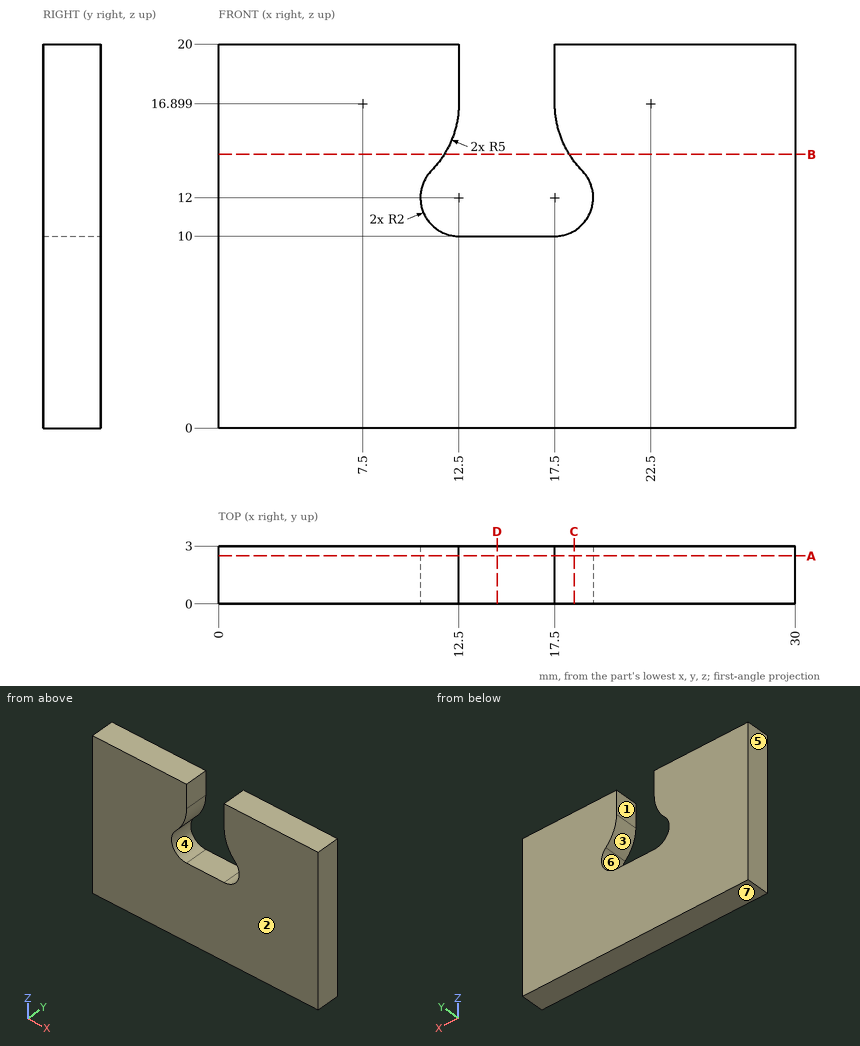
Print and shaded views of the part. All mm, measured from the part's lowest x, y and z. A direction names the side the tool comes from. Round coordinates to 2 decimals unless told otherwise and drop trailing zeros. Write each loop counter-clockwise with the first axis right and the second up, starting at its lowest first coordinate (ties: lowest second). Pieces come first, ordered by that corner, then holes. Notation, with made-up numbers: (2.5, -34) -> (12.5, -34) arc R24 cw to (12.5, -6) -> close; hole circle Ø10 at (39, 69.5). An arc over 180 degrees is marked (long way). Return JSON: item names as keys, results as strings. Group by question number.
Q1. Saw through at C-C on x = 18.5. Write the cut outline in (y, z), plus the area to 3 significant figures.
Q2. Pin check, flat tip, straight feed: pin 1 (4 mm diameter, centred on x = 13.5, z = 5, fed in from -Y). Stop position of the tip, or through.
Q3. Probe L1, parallel to X at y = 2.95, z = 18; L2, parallel to Z at x = 15.5, y = 2.3; L3, parallel to X at y = 1.4, z = 14.5. List the from-to ranges inside material, lowest first. Write a range as [from, to].
Q4. Saw through at D-D on x = 14.5. Write the cut outline in (y, z).
Q5. Mould opens along X. For the marked faces 4, 5, 6 and 7 say: pulls with the +X half, pulls with the -X half, needs draft (parallel to the pull), parting line crosses it, or undercut.
Q6. Saw through at A-A on y = 2.5. Write the cut outline in (x, z).
Q7. Which spindle directions (+Z, -Z, +X, -X, +Y, -Y) get a long thin tool onto all of the face, cutting with end or side? Do the marked faces 1, 2 and 3. Say none if no direction does.
Q8. Saw through at B-B on z = 14.25. Write the cut outline in (x, y), plus the area to 3 significant figures.
Answer:
{
 "1": {"outline": "(0, 0) -> (3, 0) -> (3, 10.27) -> (0, 10.27) -> close; (0, 13.9) -> (3, 13.9) -> (3, 20) -> (0, 20) -> close", "area": "49.1 mm2"},
 "2": {"pin 1": "y = 0"},
 "3": {"L1": "[0, 12.5], [17.5, 30]", "L2": "[0, 10]", "L3": "[0, 11.89], [18.11, 30]"},
 "4": {"outline": "(0, 0) -> (3, 0) -> (3, 10) -> (0, 10) -> close"},
 "5": {"face 4": "undercut", "face 5": "pulls with the -X half", "face 6": "undercut", "face 7": "needs draft"},
 "6": {"outline": "(0, 0) -> (30, 0) -> (30, 20) -> (17.5, 20) -> (17.5, 16.9) arc R5 ccw to (18.93, 13.4) arc R2 cw to (17.5, 10) -> (12.5, 10) arc R2 cw to (11.07, 13.4) arc R5 ccw to (12.5, 16.9) -> (12.5, 20) -> (0, 20) -> close"},
 "7": {"face 1": "+Z, +Y, -Y", "face 2": "+Z, -Z, +X, -X, -Y", "face 3": "+Y, -Y"},
 "8": {"outline": "(0, 0) -> (11.74, 0) -> (11.74, 3) -> (0, 3) -> close; (18.26, 0) -> (30, 0) -> (30, 3) -> (18.26, 3) -> close", "area": "70.4 mm2"}
}
